from build123d import *

# Parameters (mm, degrees)
F1_DEPTH = 27.178
F2_SIZE2 = 34.786244
F2_SIZE  = 27.17799


# Not quite as in the source:
# - a fillet or chamfer is up to 0.001 mm smaller than in the source, because OpenCascade refuses the exact size


with BuildPart() as f1:
    # F0 (on Top) → F1 (new body)
    with BuildSketch(Plane.XY):
        Polygon((-34.96010078, -25.4), (13.3535702478, -41.0980633142), (43.2130610643, 0), (13.3535702478, 41.0980633142), (-34.96010078, 25.4), align=None)
    extrude(amount=F1_DEPTH)

    # F2 (size 27.178 and 34.7862536797 in the source; OpenCascade refuses exactly that, so slightly less here)
    f2_edges = [f1.edges().sort_by_distance(p)[0] for p in [
        (28.283316, -20.549032, 27.178),
        (-10.803265, 33.249032, 27.178),
        (-34.960101, 0, 27.178),
        (-10.803265, -33.249032, 27.178),
        (28.283316, 20.549032, 27.178),
    ]]
    chamfer(f2_edges, length=F2_SIZE, length2=F2_SIZE2)


solid = f1.part
Model file for the job. Use its own axes, mm. Coordinates: 2 decimals unless noted, no trailing zeros. Order: outer loops, then holes, each group sorted by start corner. A loop starts at its lowest first (then second) coordinate and runs counter-clockwise, first axis right, second up. Notation, with made-up numbers: (22, 62.25) -> (36, 62.25) arc R17 ccw to (36, 68.25) -> close; hole circle Ø1 at (2.25, 71.5). An arc over 180 degrees is marked (long way). Return JSON: item names as keys, results as strings. Group by question number.
Item 1: Wall check: line 1 along Z through (x, y) = (15, 33); line 2 along Z through (x, y) = (20, -29); line 3 along Y through (x, z) = (-3, 24.5). Give the ranges that are in metal, low to high. Write a range as [from, to].
Item 2: Flat gauge pins, fed straight in: P1, Ø6, axis at x = -16.5, z = 6, coming from the +Y side; P2, Ø5, axis at y = -11, z = 9, coming from the -X side; P3, Ø8, axis at y = -13.5, z = 19, coming from the +X side. Where does each tip first touch, or does it go through?
Item 3: Saw through at C-C on z = 14.75. Write the cut outline in (x, y).
Values found:
{
 "1": {"line 1": "z = [0, 2.68]", "line 2": "z = [0, 1.35]", "line 3": "y = [-2.81, 2.81]"},
 "2": {"P1": "stops at y = 27.48", "P2": "stops at x = -26.64", "P3": "stops at x = 10.31"},
 "3": {"outline": "(-16.08, -11.68) -> (6.14, -18.9) -> (19.88, 0) -> (6.14, 18.9) -> (-16.08, 11.68) -> close"}
}
